Read the model definition and answer for the solid it produces. Units are mm, in the model's axes. Face numbers are marked on the shaded views. A direction names the side the tool comes from. Round coordinates to 2 decimals unless told otherwise and drop trailing zeros. Loops run counter-clockwise (first coordinate to the right, second up) from the corner with the lowest first, then second, coordinate; pieces in that order, holes last. Notation, with made-up numbers: (33, 9) -> (41, 9) arc R21 cw to (41, 37) -> close; hole circle Ø11 at (35.25, 14). An arc over 180 degrees is marked (long way). Put each result on its own line as item: value.
from build123d import *

# Parameters (mm, degrees)
CROQUIS1_R              = 4.05
SALIENTE_EXTRUIR2_DEPTH = 40
SALIENTE_EXTRUIR3_DEPTH = 3
CROQUIS4_R              = 10
CORTAR_EXTRUIR2_DEPTH   = 86


with BuildPart() as part:
    # Croquis1 → Saliente-Extruir2 (new body)
    with BuildSketch(Plane.XY):
        Polygon((42, 12.5), (-42, 12.5), (-42, -12.5), (-21.75, -12.5), (-21.75, 7.5), (21.75, 7.5), (21.75, -12.5), (42, -12.5), align=None)
        with Locations((-31.902194282, -2.5)):
            Circle(CROQUIS1_R, mode=Mode.SUBTRACT)
        with Locations((32.097805718, -2.5)):
            Circle(CROQUIS1_R, mode=Mode.SUBTRACT)
    extrude(amount=-SALIENTE_EXTRUIR2_DEPTH)

    # Croquis3 → Saliente-Extruir3 (add)
    with BuildSketch(Plane(origin=(40, 0, 0), x_dir=(0, 0, -1), z_dir=(1, 0, 0))):
        Polygon((30, 52.5), (40, 43.5), (40, -12.5), (0, -12.5), (0, 43.5), (10, 52.5), align=None)
    extrude(amount=SALIENTE_EXTRUIR3_DEPTH)

    # Croquis4 → Cortar-Extruir2 (cut, through all)
    with BuildSketch(Plane(origin=(43, 0, 0), x_dir=(0, 0, -1), z_dir=(1, 0, 0))):
        with Locations((20, 32.5)):
            Circle(CROQUIS4_R)
    extrude(amount=-CORTAR_EXTRUIR2_DEPTH, mode=Mode.SUBTRACT)


solid = part.part
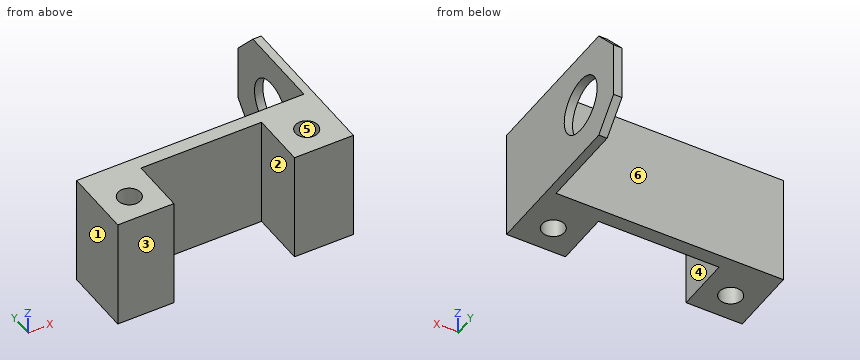
Item 1: The part is cut by section B-B (y = -2.5). Determine the outline of the cut face in (x, z).
Derived:
outline: (-42, -40) -> (-35.95, -40) -> (-35.95, 0) -> (-42, 0) -> close; (-27.85, -40) -> (-21.75, -40) -> (-21.75, 0) -> (-27.85, 0) -> close; (21.75, -40) -> (28.05, -40) -> (28.05, 0) -> (21.75, 0) -> close; (36.15, -40) -> (43, -40) -> (43, 0) -> (36.15, 0) -> close
Item 2: Find the intervals of material crossed by line 1 along X through (y, z) = (-2, -11); line 2 along Y through (x, z) = (41.25, -20); line 3 along X through (y, z) = (24, -14), in increasing order.
Derived:
line 1: x = -42 to -35.92, -27.88 to -21.75, 21.75 to 28.08, 36.12 to 43
line 2: y = -12.5 to 22.5, 42.5 to 52.5
line 3: x = 40 to 43
Item 3: The part is cut by section C-C (z = -34.5). Determine the outline of the cut face in (x, y).
Derived:
outline: (-42, -12.5) -> (-21.75, -12.5) -> (-21.75, 7.5) -> (21.75, 7.5) -> (21.75, -12.5) -> (43, -12.5) -> (43, 48.45) -> (40, 48.45) -> (40, 12.5) -> (-42, 12.5) -> close; hole circle Ø8.1 at (-31.9, -2.5); hole circle Ø8.1 at (32.1, -2.5)
Item 4: Which of the six approach directions +Z, -Z, +X, -X, +Y, -Y give full straight-line access (tool end or side, diameter ignored) to the marked faces 4, 5 and 6?
Derived:
face 4: +Z, -Z, -Y
face 5: +Z, -Z
face 6: +Z, -Z, -X, +Y
Item 5: The part is cut by section A-A (z = -20). Determine the outline of the cut face in (x, y), then the cut area to 3 significant figures.
Derived:
outline: (-42, -12.5) -> (-21.75, -12.5) -> (-21.75, 7.5) -> (21.75, 7.5) -> (21.75, -12.5) -> (43, -12.5) -> (43, 22.5) -> (40, 22.5) -> (40, 12.5) -> (-42, 12.5) -> close; (40, 42.5) -> (43, 42.5) -> (43, 52.5) -> (40, 52.5) -> close; hole circle Ø8.1 at (-31.9, -2.5); hole circle Ø8.1 at (32.1, -2.5)
area: 1,210 mm^2
Item 6: The part is cut by section D-D (y = 32.5). Determine the outline of the cut face in (x, z).
Derived:
outline: (40, -40) -> (43, -40) -> (43, -30) -> (40, -30) -> close; (40, -10) -> (43, -10) -> (43, 0) -> (40, 0) -> close
Item 7: For a pull along X with two mould halves and no side action, classify the marked faces 1, 2 and 3 as pulls with the +X half, pulls with the -X half, needs draft (parallel to the pull), parting line crosses it, or undercut.
Derived:
face 1: pulls with the -X half
face 2: undercut
face 3: needs draft
Item 8: Flat-ended cylindrical pins translate along their axes: pin 1 Ø3 at (x, z) = (-15, -5.5) entering from +Y; pin 2 Ø13 at (x, y) = (-31.9, -2.5) entering from +Z; pin 3 Ø3 at (y, z) = (23, -18.5) entering from -X; pin 4 Ø20 at (x, z) = (4, -26) entering from -Y. Find the tip coordinate at first contact, or state that the pin passes through.
Derived:
pin 1: stops at y = 12.5
pin 2: stops at z = 0
pin 3: stops at x = 40
pin 4: stops at y = 7.5
